The listing builds one solid part. Answer for the finished solid, in the listing's coordinates (mm). Coordinates: 2 decimals unless noted, no trailing zeros. Write each loop counter-clockwise with the first axis right and the second up, starting at its lowest first coordinate (ties: lowest second). Pieces come first, ordered by that corner, then holes. Notation, with made-up numbers: M 74.5,70.5 L 90.5,70.5 A26 cw 90.5,86.5 Z; hole C -8.75,49 d4. An arc over 180 degrees is marked long. Answer as a JSON object with one key per item and string values. Group by question number.
from build123d import *

# Parameters (mm, degrees)
BOSS_EXTRUDE1_DEPTH = 1.5
SKETCH2_R           = 0.5
CUT_EXTRUDE1_DEPTH  = 88.618719461
FILLET1_R           = 0.5


with BuildPart() as part:
    # Sketch1 → Boss-Extrude1 (new, symmetric)
    with BuildSketch(Plane.XY):
        Polygon((65, -3), (65, 0), (75, 0), (75, -19.1), (72, -19.1), (72, -29.1), (75, -29.1), (75, -45.2), (-75, -45.2), (-75, -29.1), (-72, -29.1), (-72, -19.1), (-75, -19.1), (-75, 0), (-65, 0), (-65, -3), (-55, -3), (-55, 0), (-35, 0), (-35, -3), (-25, -3), (-25, 0), (-5, 0), (-5, -3), (5, -3), (5, 0), (25, 0), (25, -3), (35, -3), (35, 0), (55, 0), (55, -3), align=None)
    extrude(amount=BOSS_EXTRUDE1_DEPTH, both=True)

    # Sketch2 → Cut-Extrude1 (cut, through all)
    with BuildSketch(Plane.XY.offset(1.5)):
        with Locations((-72, -29.1)):
            Circle(SKETCH2_R)
        with Locations((-72, -19.1)):
            Circle(SKETCH2_R)
        with Locations((-65, -3)):
            Circle(SKETCH2_R)
        with Locations((-55, -3)):
            Circle(SKETCH2_R)
        with Locations((-35, -3)):
            Circle(SKETCH2_R)
        with Locations((-25, -3)):
            Circle(SKETCH2_R)
        with Locations((-5, -3)):
            Circle(SKETCH2_R)
        with Locations((5, -3)):
            Circle(SKETCH2_R)
        with Locations((25, -3)):
            Circle(SKETCH2_R)
        with Locations((35, -3)):
            Circle(SKETCH2_R)
        with Locations((55, -3)):
            Circle(SKETCH2_R)
        with Locations((65, -3)):
            Circle(SKETCH2_R)
        with Locations((72, -19.1)):
            Circle(SKETCH2_R)
        with Locations((72, -29.1)):
            Circle(SKETCH2_R)
    extrude(amount=-CUT_EXTRUDE1_DEPTH, mode=Mode.SUBTRACT)

    # Fillet1
    fillet1_edges = [part.edges().sort_by_distance(p)[0] for p in [
        (72.5, -29.1, 0),
        (72, -28.6, 0),
        (72, -19.6, 0),
        (72.5, -19.1, 0),
        (65, -2.5, 0),
        (64.5, -3, 0),
        (55.5, -3, 0),
        (55, -2.5, 0),
        (35, -2.5, 0),
        (34.5, -3, 0),
        (25.5, -3, 0),
        (25, -2.5, 0),
        (5, -2.5, 0),
        (4.5, -3, 0),
        (-4.5, -3, 0),
        (-5, -2.5, 0),
        (-25, -2.5, 0),
        (-25.5, -3, 0),
        (-34.5, -3, 0),
        (-35, -2.5, 0),
        (-55, -2.5, 0),
        (-55.5, -3, 0),
        (-64.5, -3, 0),
        (-65, -2.5, 0),
        (-72.5, -19.1, 0),
        (-72, -19.6, 0),
        (-72, -28.6, 0),
        (-72.5, -29.1, 0),
    ]]
    fillet(fillet1_edges, radius=FILLET1_R)


solid = part.part
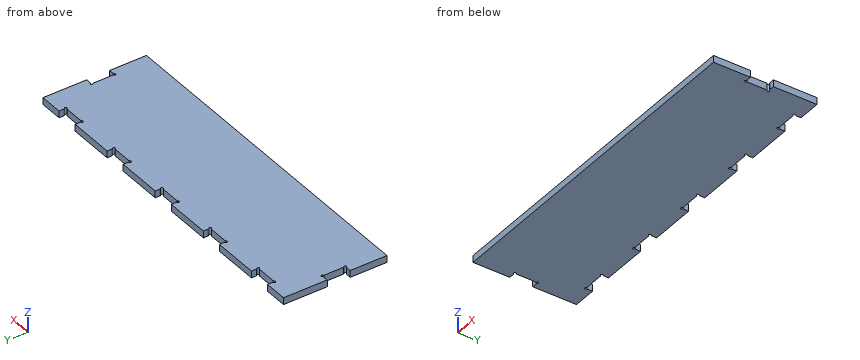
Item 1: Consider L1, parallel to X at y = -1.5, z = 0.5; L2, parallel to Y at x = -4, z = -1.2; L3, parallel to X at y = -20.5, z = 0. Determine where each line is inside the solid, lowest interval first. Write a range as from..to.
Item 2: A cutting plane is placed at A-A, the plane y = -25. Write down the section's boundary in (x, z).
Item 3: A flat-ended cylindrical pin translates along its axis: pin 1 Ø1.5 at (x, z) = (-31.5, -0.5) entering from +Y. Find the tip coordinate at first contact, or state that the pin passes through.
Answer:
{
 "1": {"L1": "-75..-65, -55..-35, -25..-5, 5..25, 35..55, 65..75", "L2": "-45.2..-3", "L3": "-72..72"},
 "2": {"outline": "M -72,-1.5 L 72,-1.5 L 72,1.5 L -72,1.5 Z"},
 "3": {"pin 1": "y = -3"}
}
